Input: part model. Units: mm. Frame: model coordinates. Coordinates: 2 decimals unless noted, no trailing zeros. Loops run counter-clockwise (first coordinate to the right, second up) from the corner with the lowest first, then second, coordinate; pieces in that order, holes last.
Item 1: Section D-D on x = 4. Return loops of the section in (y, z).
Item 2: Section A-A on y = -3. Return loops of the section in (x, z).
Item 3: Section C-C on z = -120.5. Return loops of the section in (x, y).
Item 4: Pull-direction query (X, two-part tool) for faces 1 (the cylindrical face through (5.723, 1.802, -68.28)), 2 (the flat face through (0, 0, 0)), 3 (the cylindrical face through (-0.088, -0.084, -122.498)); classes: released by +X, released by -X, zero draft, split by the parting line, or undercut.
Item 5: Contact query for flat-ended pins moving along their axis: P1, Ø3, axis at y = 4.5, z = -28.5, coming from the -X side; P2, Ø6, axis at x = -3.5, z = -79.5, coming from the -Y side; P3, Ø6, axis at x = 4, z = -27, coming from the +Y side. Output: stop coordinate, or through.
Item 6: Section B-B on z = -31.5. Return loops of the section in (x, y), and give its area (3 significant figures).
Item 7: Ray query, line 1 along Z through (x, y) = (0, 0.5); line 2 along X through (y, z) = (0.75, -120.5); line 3 along Z through (x, y) = (-1.75, 1.75). Return the intervals inside material, ascending.
Autodesk Inventor part; units mm, degrees
ref_plane "YZ Plane" through (0, 0, 0) normal (1, 0, 0) x (0, 1, 0)
ref_plane "XZ Plane" through (0, 0, 0) normal (0, 1, 0) x (-1, 0, 0)
ref_plane "XY Plane" through (0, 0, 0) normal (0, 0, 1) x (1, 0, 0)
sketch "スケッチ1" plane through (0, 0, 0) normal (0, 0, 1) x (1, 0, 0)
  circle A0 centre (0, 0) radius 6
  dimension "d0" = 12
extrude "押し出し1" add sketch "スケッチ1" against normal blind 138.5
sketch "スケッチ2" plane through (0, 0, 0) normal (0, 1, 0) x (-1, 0, 0)
  line L0 (0, 0) -> (0, -138.5)
  line L1 (-6, -138.5) -> (6, -138.5)
  line L2 (6, 0) -> (-6, 0)
  point P0 (0, -3)
  point P1 (0, -53)
  point P2 (0, -64)
  point P3 (0, -120.5)
  point P4 (0, -135.5)
  dimension "d3" = 3
  dimension "d4" = 53
  dimension "d5" = 64
  dimension "d6" = 3
  dimension "d7" = 18
hole "穴1" at (0, 0, -3) at (0, 0, -64) at (0, 0, -135.5) direction (0, -1, 0) diameter 2 end through all both
hole "穴2" at (0, 0, -53) at (0, 0, -120.5) direction (0, -1, 0) diameter 4 end through all both
properties part number "ローラー_軸"
Results found:
1. outline: (-4.47, -138.5) - (4.47, -138.5) - (4.47, 0) - (-4.47, 0) - close
2. outline: (-5.2, -138.5) - (5.2, -138.5) - (5.2, 0) - (-5.2, 0) - close; hole circle Ø4 at (0, -120.5); hole circle Ø4 at (0, -53); hole circle Ø2 at (0, -135.5); hole circle Ø2 at (0, -64); hole circle Ø2 at (0, -3)
3. outline: (-2, -5.66) - (-2, 5.66) arc R6 ccw to start; (2, -5.66) arc R6 ccw to (2, 5.66) - close
4. face 1: split by the parting line
4. face 2: zero draft
4. face 3: undercut
5. P1: stops at x = -5.2
5. P2: stops at y = -5.98
5. P3: stops at y = 5.92
6. outline: circle Ø12 at (0, 0)
6. area: 113 mm2
7. line 1: z = -138.5 to -136.5, -134.5 to -122.5, -118.5 to -65, -63 to -55, -51 to -4, -2 to 0
7. line 2: x = -5.95 to -2, 2 to 5.95
7. line 3: z = -138.5 to -121.47, -119.53 to -53.97, -52.03 to 0
